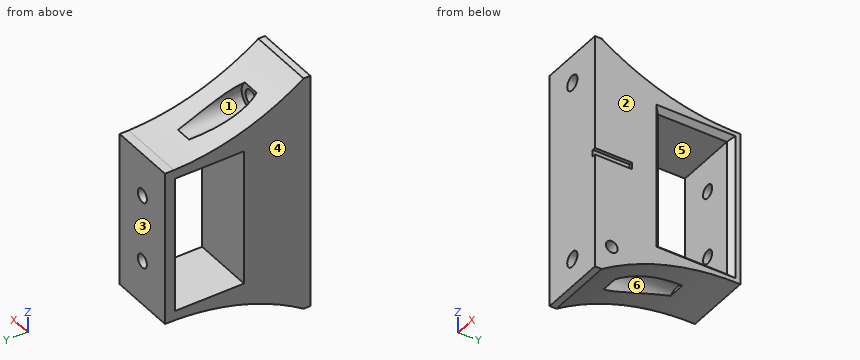
Autodesk Inventor part; units mm, degrees
ref_plane "YZ Plane" through (0, 0, 0) normal (1, 0, 0) x (0, 1, 0)
ref_plane "XZ Plane" through (0, 0, 0) normal (0, 1, 0) x (-1, 0, 0)
ref_plane "XY Plane" through (0, 0, 0) normal (0, 0, 1) x (1, 0, 0)
sketch "Sketch1" plane through (0, 0, 0) normal (1, 0, 0) x (0, 1, 0)
  line L0 (0, 0) -> (0, -35.25)
  line L1 (0, -35.25) -> (2, -35.25)
  line L2 (19.75, 20.25) -> (40.25, 20.25)
  line L3 (40.25, 20.25) -> (40.25, -20.25)
  line L4 (40.25, -20.25) -> (19.75, -20.25)
  line L5 (19.75, -20.25) -> (19.75, 20.25)
  line L6 (19.75, 20.25) -> (40.25, -20.25) construction
  line L7 (40.25, 20.25) -> (19.75, -20.25) construction
  line L8 (16.75, 23) -> (43.25, 23)
  line L9 (43.25, 23) -> (43.25, -23)
  line L10 (43.25, -23) -> (16.75, -23)
  line L11 (16.75, -23) -> (16.75, 23)
  line L12 (16.75, 23) -> (43.25, -23) construction
  line L13 (43.25, 23) -> (16.75, -23) construction
  line L14 (0, 0) -> (0, 35.25)
  line L15 (0, 35.25) -> (2, 35.25)
  arc A0 (2, 35.25) -> (43.25, 23) centre (41.9161, 94.0847) ccw
  arc A1 (43.25, -23) -> (2, -35.25) centre (42.6775, -96.6486) ccw
  line L16 (-8.65, 0) -> (51.9, 0)
  point P0 (20, 0)
  point P1 (40.1, 0)
  point P2 (30, 0)
  point P3 (30, 23)
  point P4 (30.2, -23)
  point P5 (30, 0)
  dimension "d0" = 35.25
  dimension "d1" = 2
  dimension "d2" = 20
  dimension "d4" = 20.5
  dimension "d5" = 40.5
  dimension "d6" = 46
  dimension "d7" = 26.5
  dimension "d8" = 35.25
extrude "Extrusion1" add sketch "Sketch1" along normal blind 20 contours L10 L11 L16 L5 L4 L3 L9 | L16 L11 L10 A1 L1 L0 | L14 L15 A0 L8 L11 L16 | L11 L8 A0 L9 L16 L3 L2 L5 | L8 A0
sketch "Sketch2" plane through (0, 43.25, 23) normal (0, 1, 0) x (1, 0, 0)
  line L0 (0, 46) -> (0, 0)
  line L1 (0, 0) -> (20, 0)
  line L2 (20, 46) -> (20, 0)
  line L3 (0, 46) -> (20, 46)
  line L4 (0, 2.75) -> (20, 2.75)
  line L5 (0, 2.75) -> (20, 2.75)
  point P0 (0, 23)
  point P1 (10, 12.8)
  point P2 (10, 32.8)
  dimension "d33" = 20
  dimension "d34" = 10.05
hole "Hole1" at (10, 43.25, 10.2) at (10, 43.25, -9.8) direction (0, -1, 0) diameter 4 end up to surface
ref_plane "Work Plane1" through (0, 11, -35.25) normal (0, -1, 0) x (1, 0, 0)
sketch "Sketch3" plane through (0, 11, -35.25) normal (0, -1, 0) x (1, 0, 0)
  circle A0 centre (10, 45.45) radius 2
  line L0 (0, 12.25) -> (0, 58.25)
  line L1 (0, 58.25) -> (20, 58.25)
  line L2 (20, 12.25) -> (20, 58.25)
  line L3 (0, 12.25) -> (20, 12.25)
  line L4 (0, 55.5) -> (0, 15)
  line L5 (0, 55.5) -> (20, 55.5)
  line L6 (20, 15) -> (20, 55.5)
  line L7 (0, 15) -> (20, 15)
  circle A1 centre (10, 62.25) radius 4
  circle A2 centre (10, 8.25) radius 4
  point P0 (0, 35.25)
  dimension "d19" = 4
  dimension "d20" = 4
  dimension "d30" = 8
  dimension "d31" = 8
extrude "Extrusion2" cut sketch "Sketch3" against normal blind 20 contours A1 | A2
hole "Hole2" at (10, 11, 27) at (10, 11, -27) direction (0, -1, 0) diameter 4.5 end through all
chamfer "Chamfer1" distance 1.5 angle 45 4 edges at (20, 40.25, 0) (20, 30, 20.25) (20, 19.75, 0) (20, 30, -20.25)
sketch "Sketch4" plane through (20, 0, 0) normal (1, 0, 0) x (0, 0, -1)
  line L0 (0, -8.65) -> (0, 51.9)
  line L1 (-35.25, 0) -> (35.25, 0)
  line L2 (0, 0) -> (-1, 0)
  line L3 (-1, 0) -> (-1, 11)
  line L4 (-1, 11) -> (0, 11)
  line L5 (0, 11) -> (0, 0)
  line L6 (0, 11) -> (1, 11)
  line L7 (1, 11) -> (1, 0)
  line L8 (1, 0) -> (0, 0)
  line L9 (0, 0) -> (0, 11)
  dimension "d51" = 1
  dimension "d52" = 1
extrude "Extrusion3" cut sketch "Sketch4" against normal blind 1
sketch "Sketch5" plane through (20, 0, 0) normal (1, 0, 0) x (0, 0, -1)
  line L0 (0, 0) -> (35.25, 0)
  line L1 (35.25, 0) -> (35.25, 2)
  point P0 (27.25, 5)
  dimension "d42" = 5
  dimension "d43" = 8
hole "Hole3" at (20, 5, -27.25) direction (-1, 0, 0) diameter 3.5 depth 5
equation "\"d8\" = d0"
equation "\"d31\" = d30"
equation "\"d52\" = d51"
properties part number "espaceur_20mm_v4"
For this review, take the finished solid that the model builds, in its own axes (mm). Face numbers are marked on the shaded views. A direction names the side the tool comes from. Round coordinates to 2 decimals unless told otherwise and drop trailing zeros. Loops run counter-clockwise (first coordinate to the right, second up) from the corner with the lowest first, then second, coordinate; pieces in that order, holes last. Notation, with made-up numbers: (18, -24.5) - (43, -24.5) arc R25 ccw to (43, 4.5) - close; hole circle Ø6 at (-5, 17). An arc over 180 degrees is marked (long way). Put each result on its own line as item: value. Start each with the question number.
1. Mouldability with a two-part tool opening along X and no side actions: class the marked faces 1, 2 and 3 as +X half, -X half, draft (parallel to the pull), parting line (faces both ways), or undercut.
2. Consider section B-B on x = 2.75. State the section outline as (y, z) points.
3. Consider section D-D on y = 33. State the section outline as (x, z) points.
4. Consider section C-C on x = 17. State the section outline as (y, z) points.
5. For probe 1 along Y at (x, z) = (1.5, -11); probe 2 along X at (y, z) = (17.25, -27); probe 3 along Z at (x, y) = (10, 42.35), list the stretches that pass through material, from the lowest coordinate up. Write a range as [from, to].
6. For the marked faces 4, 5 and 6, list the 3-axis set-ups (+Z, -Z, +X, -X, +Y, -Y) from which the entire face can be reached by the end or side of a thin tool; tool diameter is ignored.
7. Insertion check: P1, Ø2, axis at x = 7.5, z = -27, coming from the +Y side; P2, Ø3, axis at x = 3, y = 17, coming from the -Z side; P3, Ø6, axis at y = 23, z = 15, coming from the -X side; P4, Ø1.1, axis at x = 19.5, y = 5.5, coming from the -Z side. Each pin has a flat end and moves straight along its axis. Give the tip position at first contact, or say it passes through.
8. Consider section A-A on z = 13.5. State the section outline as (x, y) points.
Result sheet:
1. face 1: undercut
1. face 2: +X half
1. face 3: draft
2. outline: (0, -35.25) - (2, -35.25) arc R73.65 cw to (43.25, -23) - (43.25, 23) - (40.58, 23) arc R71.1 cw to (2, 35.25) - (0, 35.25) - close; hole (19.75, -20.25) - (40.25, -20.25) - (40.25, 20.25) - (19.75, 20.25) - close
3. outline: (0, -23.64) - (20, -23.64) - (20, -21.75) - (18.5, -20.25) - (0, -20.25) - close; (0, 20.25) - (18.5, 20.25) - (20, 21.75) - (20, 23.55) - (0, 23.55) - close
4. outline: (0, -35.25) - (2, -35.25) arc R73.65 cw to (43.25, -23) - (43.25, 23) - (40.58, 23) arc R71.1 cw to (2, 35.25) - (0, 35.25) - close; hole circle Ø3.5 at (5, -27.25); hole (19.75, -20.25) - (40.25, -20.25) - (40.25, 20.25) - (19.75, 20.25) - close
5. probe 1: [0, 19.75], [40.25, 43.25]
5. probe 2: [0, 6], [14, 20]
5. probe 3: [-23, -11.8], [-7.8, 8.2], [12.2, 23]
6. face 4: +Z, -Z, -X, +Y, -Y
6. face 5: +X, -X
6. face 6: none
7. P1: y = 11
7. P2: z = -28.2
7. P3: through
7. P4: z = -33.39
8. outline: (0, 0) - (20, 0) - (20, 18.25) - (18.5, 19.75) - (0, 19.75) - close; (0, 40.25) - (18.5, 40.25) - (20, 41.75) - (20, 43.25) - (0, 43.25) - close
